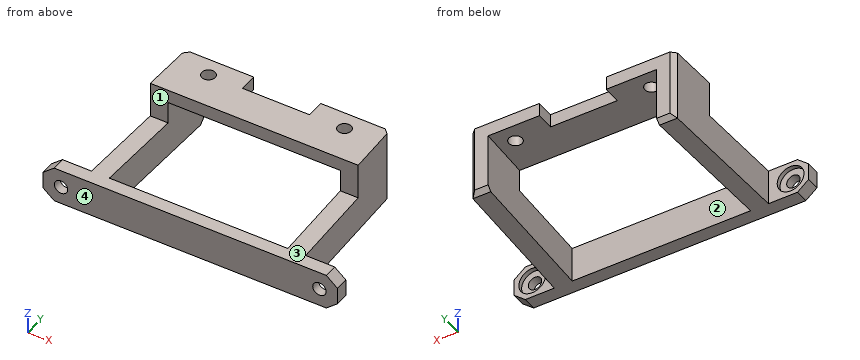
from build123d import *
from OCP.BRepFilletAPI import BRepFilletAPI_MakeChamfer

# Parameters (mm, degrees)
SKETCH1_W           = 66
SKETCH1_H           = 8
SKETCH1_R           = 1.5
BOSS_EXTRUDE1_DEPTH = 3
BOSS_EXTRUDE4_DEPTH = 8
BOSS_EXTRUDE6_DEPTH = 8
SKETCH7_R           = 3
CUT_EXTRUDE1_DEPTH  = 1
SKETCH8_W           = 15
SKETCH8_H           = 4
CUT_EXTRUDE2_DEPTH  = 8
CUT_EXTRUDE3_DEPTH  = 5
CHAMFER2_SIZE       = 1
CHAMFER2_SIZE2      = 1.036815955
SKETCH10_R          = 1.5
CUT_EXTRUDE4_DEPTH  = 3
CUT_EXTRUDE5_DEPTH  = 3


with BuildPart() as part:
    # Sketch1 → Boss-Extrude1 (new body)
    with BuildSketch(Plane(origin=(0, 0, 0), x_dir=(1, 0, 0), z_dir=(0, 1, 0))):
        Rectangle(SKETCH1_W, SKETCH1_H)
        with Locations(Location((-28.953010595, 0, 0), (0, 0, 270))):
            Circle(SKETCH1_R, mode=Mode.SUBTRACT)
        with Locations(Location((28.953010595, 0, 0), (0, 0, 270))):
            Circle(SKETCH1_R, mode=Mode.SUBTRACT)
    extrude(amount=BOSS_EXTRUDE1_DEPTH)

    # Sketch4 → Boss-Extrude4 (add)
    with BuildSketch(Plane.XY.offset(4)):
        Polygon((-24, 3), (-22.882535376, 35), (-18.880097199, 35), (-19.997561823, 3), align=None)
    boss_extrude4 = extrude(amount=-BOSS_EXTRUDE4_DEPTH)

    # Mirror1: Boss-Extrude4 across plane
    add(boss_extrude4.mirror(Plane(origin=(0, 0, 0), x_dir=(0, 0, 1), z_dir=(1, 0, 0))))

    # Sketch6 → Boss-Extrude6 (add)
    with BuildSketch(Plane.XY.offset(4)):
        Polygon((-22.882535376, 35), (22.882535376, 35), (23.30158461, 23), (-23.30158461, 23), align=None)
    extrude(amount=BOSS_EXTRUDE6_DEPTH)

    # Sketch7 → Cut-Extrude1 (cut)
    with BuildSketch(Plane(origin=(0, 3, 0), x_dir=(1, 0, 0), z_dir=(0, 1, 0))):
        with Locations(Location((-28.953010595, 0, 0), (0, 0, 270))):
            Circle(SKETCH7_R)
        with Locations(Location((28.953010595, 0, 0), (0, 0, 270))):
            Circle(SKETCH7_R)
    extrude(amount=-CUT_EXTRUDE1_DEPTH, mode=Mode.SUBTRACT)

    # Sketch8 → Cut-Extrude2 (cut)
    with BuildSketch(Plane.XY.offset(12)):
        with Locations((-0.1, 33)):
            Rectangle(SKETCH8_W, SKETCH8_H)
    extrude(amount=-CUT_EXTRUDE2_DEPTH, mode=Mode.SUBTRACT)

    # Sketch9 → Cut-Extrude3 (cut)
    with BuildSketch(Plane(origin=(0, 0, 4), x_dir=(-1, 0, 0), z_dir=(0, 0, -1))):
        Polygon((-19.299146433, 23), (19.299146433, 23), (18.880097199, 35), (-18.880097199, 35), align=None)
    extrude(amount=-CUT_EXTRUDE3_DEPTH, mode=Mode.SUBTRACT)

    # Chamfer2: one chamfer whose edges measure the first distance from different faces: ONE call of the kernel's chamfer builder (chamfer() names one face for all edges)
    chamfer2_edges_1 = [part.edges().sort_by_distance(p)[0] for p in [
        (-22.882535376, 35, 4),
    ]]
    chamfer2_side_1 = [part.faces().sort_by_distance(p)[0] for p in [
        (-23.346029226, 21.727272727, 2.181818182),
    ]]
    chamfer2_edges_2 = [part.edges().sort_by_distance(p)[0] for p in [
        (-20.881316288, 35, -4),
        (20.881316288, 35, -4),
    ]]
    chamfer2_edges_3 = [part.edges().sort_by_distance(p)[0] for p in [
        (22.882535376, 35, 4),
    ]]
    chamfer2_side_3 = [part.faces().sort_by_distance(p)[0] for p in [
        (22.659890165, 35, 4),
    ]]
    chamfer2 = BRepFilletAPI_MakeChamfer(part.part.solid().wrapped)
    for e in chamfer2_edges_1:
        chamfer2.Add(CHAMFER2_SIZE, CHAMFER2_SIZE2, e.wrapped, chamfer2_side_1[0].wrapped)  # the first distance lies on this face
    for e in chamfer2_edges_2:
        chamfer2.Add(CHAMFER2_SIZE, e.wrapped)
    for e in chamfer2_edges_3:
        chamfer2.Add(CHAMFER2_SIZE, CHAMFER2_SIZE2, e.wrapped, chamfer2_side_3[0].wrapped)  # the first distance lies on this face
    add(Compound.cast(chamfer2.Shape()), mode=Mode.REPLACE)

    # Sketch10 → Cut-Extrude4 (cut)
    with BuildSketch(Plane(origin=(0, 0, 9), x_dir=(-1, 0, 0), z_dir=(0, 0, -1))):
        with Locations((-15.24, 31)):
            Circle(SKETCH10_R)
        with Locations((15.24, 31)):
            Circle(SKETCH10_R)
    extrude(amount=-CUT_EXTRUDE4_DEPTH, mode=Mode.SUBTRACT)

    # Sketch13 → Cut-Extrude5 (cut)
    with BuildSketch(Plane(origin=(0, 3, 0), x_dir=(1, 0, 0), z_dir=(0, 1, 0))):
        Polygon((-30.5, 4), (-33, 1.902250922), (-33, 4), align=None)
        Polygon((-30.5, -4), (-33, -1.902250922), (-33, -4), align=None)
        Polygon((30.5, -4), (33, -1.902250922), (33, -4), align=None)
        Polygon((30.5, 4), (33, 1.902250922), (33, 4), align=None)
    extrude(amount=-CUT_EXTRUDE5_DEPTH, mode=Mode.SUBTRACT)


solid = part.part
For this review, take the finished solid that the model builds, in its own axes (mm). Face numbers are marked on the shaded views. A direction names the side the tool comes from. Coordinates: 2 decimals unless noted, no trailing zeros. Order: outer loops, then holes, each group sorted by start corner. A loop starts at its lowest first (then second) coordinate and runs counter-clockwise, first axis right, second up. Notation, with made-up numbers: (88.5, -33) - (134.5, -33) arc R25 ccw to (134.5, -5) - close; hole circle Ø1 at (47, 40). An arc over 180 degrees is marked (long way). Answer as CSV lines item,"result". Start each with the question number.
1) To check wall thickness, follow line 1 along X through (y, z) = (2.6, 0); line 2 along X through (y, z) = (1.4, 0); line 3 along Y through (x, z) = (15.24, 10). State the ranges of each line that lie inside material, in increasing order. Write a range as [from, to].
2) Add section D-D (y = 18). State the section outline as (x, z) points.
3) Add section B-B (x = -15.24). State the section outline as (y, z) points.
4) Add section A-A (z = 6.75). State the section outline as (x, y) points.
5) Draft analysis for pull direction X (two halves, no side actions). For the marked faces 1 and 2, state which applies: +X half, -X half, draft (parallel to the pull), parting line (faces both ways), or undercut.
6) Insertion check: P1, Ø3, axis at x = -28.5, z = 0.5, coming from the +Y side; P2, Ø8, axis at y = 18.5, z = 1.5, coming from the +X side; P3, Ø1, axis at y = 11.5, z = 1.5, coming from the +X side. Each pin has a flat end and moves straight along its axis. Give the tip position at first contact, or say it passes through.
7) Add section C-C (z = 0). Count the separate pieces of the cut face and the enclosed holes in it, then the cut area to 3 significant figures.
8) Machinability: for the marked faces 3 and 4, which of the approach directions +Z, -Z, +X, -X, +Y, -Y give a long, thin tool a straight path to every point of the face, cutting with its end or side? Answer none if there is none.
Result:
1,line 1,"[-33, -31.95], [-25.95, 25.95], [31.95, 33]"
1,line 2,"[-33, -30.45], [-27.45, 27.45], [30.45, 33]"
1,line 3,"[23, 29.5], [32.5, 35]"
2,outline,"(-23.48, -4) - (-19.47, -4) - (-19.47, 4) - (-23.48, 4) - close; (19.47, -4) - (23.48, -4) - (23.48, 4) - (19.47, 4) - close"
3,outline,"(0, -4) - (3, -4) - (3, 4) - (0, 4) - close; (23, 9) - (29.5, 9) - (29.5, 12) - (23, 12) - close; (32.5, 9) - (35, 9) - (35, 12) - (32.5, 12) - close"
4,outline,"(-23.3, 23) - (-19.3, 23) - (-18.88, 35) - (-21.85, 35) - (-22.92, 34) - close; (18.88, 35) - (19.3, 23) - (23.3, 23) - (22.92, 33.96) - (21.88, 35) - close"
5,face 1,"draft"
5,face 2,"undercut"
6,P1,"y = 2"
6,P2,"x = 23.6"
6,P3,"x = 23.72"
7,separate pieces,"3"
7,enclosed holes,"0"
7,area,"429 mm^2"
8,face 3,"+Z, +X, -X, -Y"
8,face 4,"+Z, -Z, +X, -X, -Y"
